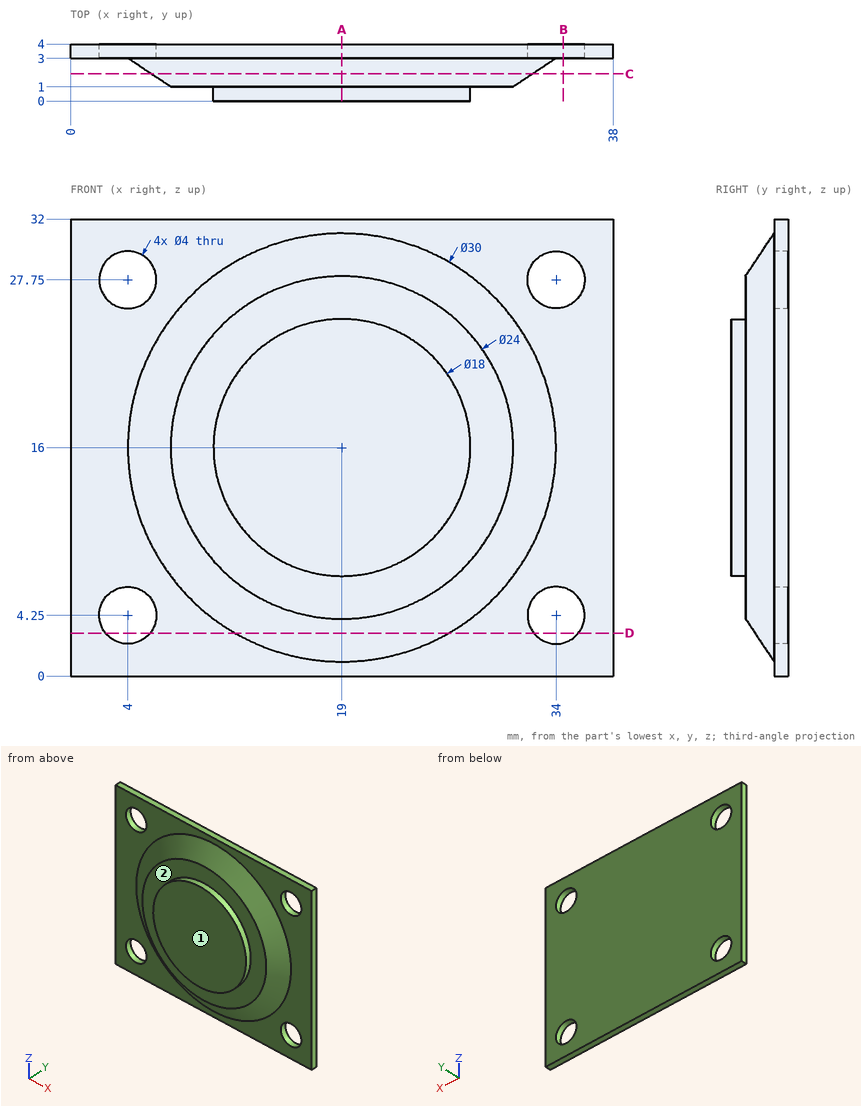
Job drawing, mm, ordinate dimensions from the low corner. One solid piece. A direction names the side the tool comes from. Round coordinates to 2 decimals unless told otherwise and drop trailing zeros. Loops run counter-clockwise (first coordinate to the right, second up) from the corner with the lowest first, then second, coordinate; pieces in that order, holes last. Notation, with made-up numbers: M -26.5,62 L 19.5,62 A11 cw 19.5,78 Z; hole C 16,-16 d10. An arc over 180 degrees is marked long. One line per question, with ' | ' between items. Start each with the question number.
Item 1: Cut at B-B, the plane x = 34.5. Write the cut outline in (y, z), plus the area to 3 significant figures.
Item 2: Cut at C-C, the plane y = 1.9. Write the cut outline in (x, z).
Item 3: Cut at A-A, the plane x = 19. Write the cut outline in (y, z), plus the area to 3 significant figures.
Item 4: Pin check, flat tips, straight feed: pin 1 Ø1 at (x, y) = (18.5, 1) entering from +Z; pin 2 Ø2.5 at (x, z) = (4, 27.75) entering from +Y; pin 3 Ø4.5 at (x, z) = (34, 4.25) entering from -Y; pin 4 Ø1 at (x, y) = (24.5, 1.5) entering from -Z. Stop position of each tip, or through.
Item 5: Cut at D-D, the plane z = 3. State how many separate pieces and enclosed holes the cut face has, plus the area to 3 significant figures.
Item 6: Wall check: line 1 (X direction, y = 3.3, z = 4.25); line 2 (Z direction, x = 4, y = 3.6); line 3 (X direction, y = 3.75, z = 3.5). Give the ranges that are in metal, low to high.
Item 7: Which spindle directions (+Z, -Z, +X, -X, +Y, -Y) get a long thin tool onto all of the face, cutting with end or side? Do the marked faces 1 and 2. Say none if no direction does.
Responses:
1) outline: M 3,0 L 4,0 L 4,2.31 L 3,2.31 Z; M 3,6.19 L 4,6.19 L 4,25.81 L 3,25.81 Z; M 3,29.69 L 4,29.69 L 4,32 L 3,32 Z | area: 24.3 mm²
2) outline: C 19,16 d26.7
3) outline: M 0,7 L 1,7 L 1,4 L 3,1 L 3,0 L 4,0 L 4,32 L 3,32 L 3,31 L 1,28 L 1,25 L 0,25 Z | area: 104 mm²
4) pin 1: stops at z = 28.74 | pin 2: passes through | pin 3: stops at y = 3 | pin 4: stops at z = 3.64
5) separate pieces: 3 | enclosed holes: 0 | area: 44.9 mm²
6) line 1: x = 0 to 2, 6 to 32, 36 to 38 | line 2: z = 0 to 2.25, 6.25 to 25.75, 29.75 to 32 | line 3: x = 0 to 2.15, 5.85 to 32.15, 35.85 to 38
7) face 1: +Z, -Z, +X, -X, -Y | face 2: -Y
